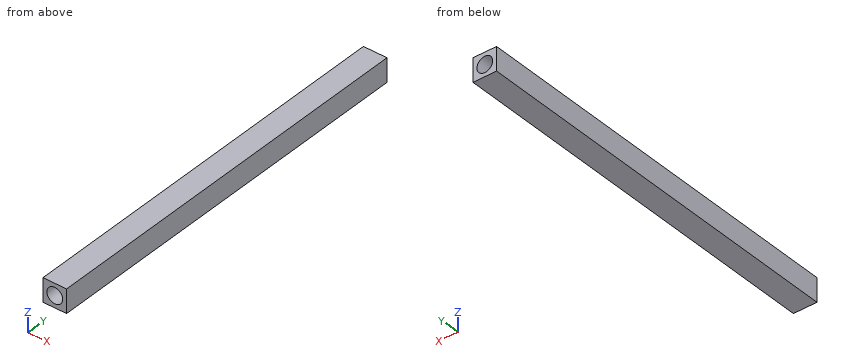
Autodesk Inventor part; units mm, degrees
ref_plane "YZ Plane" through (0, 0, 0) normal (1, 0, 0) x (0, 1, 0)
ref_plane "XZ Plane" through (0, 0, 0) normal (0, 1, 0) x (-1, 0, 0)
ref_plane "XY Plane" through (0, 0, 0) normal (0, 0, 1) x (1, 0, 0)
sketch "Sketch1" plane through (0, 0, 0) normal (0, 1, 0) x (-1, 0, 0)
  line L0 (3, 3) -> (3, -3)
  line L1 (3, -3) -> (-3, -3)
  line L2 (-3, -3) -> (-3, 3)
  line L3 (-3, 3) -> (3, 3)
  line L4 (3, 3) -> (-3, -3) construction
  line L5 (3, -3) -> (-3, 3) construction
  circle A0 centre (0, 0) radius 2
  dimension "d0" = 6
  dimension "d1" = 6
  dimension "d2" = 4
extrude "Extrusion1" add sketch "Sketch1" along normal blind 100
ref_plane "Work Plane1" through (0, 0, 3) normal (1, 0, 0) x (0, 0, -1)
properties part number "carbon_fiber_6"
The model under review builds one solid part; all positions refer to its coordinate system, in mm. Coordinates: 2 decimals unless noted, no trailing zeros. Loops run counter-clockwise (first coordinate to the right, second up) from the corner with the lowest first, then second, coordinate; pieces in that order, holes last. Notation, with made-up numbers: (-15.5, -31.75) -> (-9.5, -31.75) arc R21 cw to (-9.5, 2.25) -> close; hole circle Ø8 at (60, 66). An arc over 180 degrees is marked (long way). Use a Markdown table: item, result. Add a question column.
1. Add section B-B on z = 0. Write out the cut boundary in (x, y), plus the area to 3 significant figures.
2. To check wall thickness, follow line 1 (Z direction, x = 0, y = 60); line 2 (X direction, y = 5, z = -1); line 3 (X direction, y = 12.5, z = 1.4). State the ranges of each line that lie inside material, in increasing order.
3. Add section C-C on y = 72. Write out the cut boundary in (x, z), plus the area to 3 significant figures.
4. Add section A-A on x = 0. Write out the cut boundary in (y, z), plus the area to 3 significant figures.
Returned:
| question | item | result |
|---|---|---|
| 1 | outline | (-3, 0) -> (-2, 0) -> (-2, 100) -> (-3, 100) -> close; (2, 0) -> (3, 0) -> (3, 100) -> (2, 100) -> close |
| 1 | area | 200 mm² |
| 2 | line 1 | z = -3 to -2, 2 to 3 |
| 2 | line 2 | x = -3 to -1.73, 1.73 to 3 |
| 2 | line 3 | x = -3 to -1.43, 1.43 to 3 |
| 3 | outline | (-3, -3) -> (3, -3) -> (3, 3) -> (-3, 3) -> close; hole circle Ø4 at (0, 0) |
| 3 | area | 23.4 mm² |
| 4 | outline | (0, -3) -> (100, -3) -> (100, -2) -> (0, -2) -> close; (0, 2) -> (100, 2) -> (100, 3) -> (0, 3) -> close |
| 4 | area | 200 mm² |
